from build123d import *

# Parameters (mm, degrees)
BOSS_EXTRUDE1_DEPTH = 6
FILLET1_R           = 1
FILLET2_R           = 0.5
SKETCH2_R           = 1.6
CUT_EXTRUDE2_DEPTH  = 10


with BuildPart() as part:
    # Sketch1 → Boss-Extrude1 (new body)
    with BuildSketch(Plane(origin=(0, 41.463460463, 0), x_dir=(1, 0, 0), z_dir=(0, 1, 0))):
        with BuildLine():
            Line((26.614370899, -46.171636097), (23.614370899, -38.171636097))
            Line((23.614370899, -38.171636097), (17.614370899, -38.171636097))
            Line((17.614370899, -38.171636097), (17.614370899, -35.202564725))
            Line((17.614370899, -35.202564725), (45.614370899, -35.202564725))
            Line((45.614370899, -35.202564725), (45.614370899, -38.171636097))
            Line((45.614370899, -38.171636097), (39.614370899, -38.171636097))
            Line((39.614370899, -38.171636097), (36.614370899, -46.171636097))
            ThreePointArc((36.614370899, -46.171636097), (31.614370899, -41.171636097), (26.614370899, -46.171636097))
        make_face()
    extrude(amount=-BOSS_EXTRUDE1_DEPTH)

    # Fillet1
    fillet1_edges = [part.edges().sort_by_distance(p)[0] for p in [
        (17.614370899, 41.463460463, 36.687100411),
        (45.614370899, 41.463460463, 36.687100411),
    ]]
    fillet(fillet1_edges, radius=FILLET1_R)

    # Fillet2
    fillet2_edges = [part.edges().sort_by_distance(p)[0] for p in [
        (36.614370899, 38.463460463, 46.171636097),
        (26.614370899, 38.463460463, 46.171636097),
    ]]
    fillet(fillet2_edges, radius=FILLET2_R)

    # Sketch2 → Cut-Extrude2 (cut)
    with BuildSketch(Plane(origin=(0, 0, 35.202564725), x_dir=(-1, 0, 0), z_dir=(0, 0, -1))):
        with Locations((-20.74213752, 38.663460463)):
            Circle(SKETCH2_R)
        with Locations((-42.486604277, 38.663460463)):
            Circle(SKETCH2_R)
    extrude(amount=-CUT_EXTRUDE2_DEPTH, mode=Mode.SUBTRACT)


solid = part.part
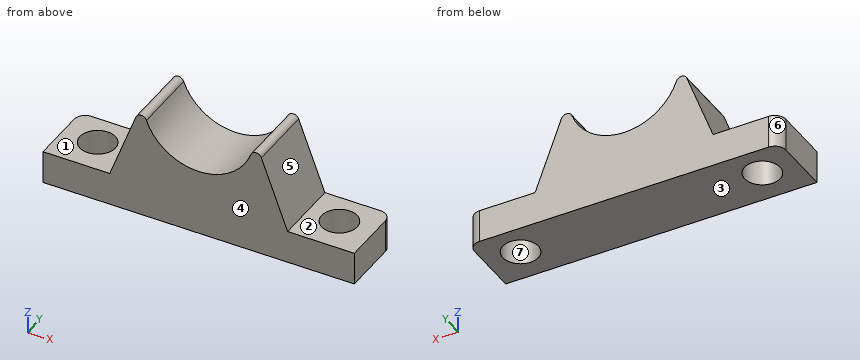
Here's how the part is built. I have some questions about the finished solid (model axes, mm). Face numbers are marked on the shaded views. A direction names the side the tool comes from. Round coordinates to 2 decimals unless told otherwise and drop trailing zeros. Write each loop counter-clockwise with the first axis right and the second up, starting at its lowest first coordinate (ties: lowest second). Pieces come first, ordered by that corner, then holes.
1. Suppose I cut it at C-C (y = 36.05). List the corners of the cut face in (x, z) for me, and give its area (3 significant figures).
2. Suppose I cut it at A-A (y = 39.55). List the corners of the cut face in (x, z) for me.
3. For the marked faces 1, 2 and 3, which set-ups out of +Z, -Z, +X, -X, +Y, -Y let a thin tool reach every point of the face, with its end or its side?
4. I need wall thicknesses on L1, parallel to X at y = 36.6, z = 42.25; L2, parallel to Y at x = 19.5, z = 37; L3, parallel to X at y = 37.95, z = 42.75. Which ranges of each line are inside material? Lowest first, please.
5. Will these pins go through, and if not, where does the flat tip stop? pin 1 Ø3 at (x, y) = (43, 38.5) entering from +Z; pin 2 Ø3 at (y, z) = (38.5, 40) entering from +X.
6. If we mould it in two halves opening along Y, with no side actions, what happens to the marked faces 4, 5, 6 and 7? For each: released by +Y, released by -Y, zero draft, split by the parting line, or undercut.
7. Suppose I cut it at B-B (x = 20.75). List the corners of the cut face in (y, z) for me, and give its area (3 significant figures).
8. Suppose I cut it at D-D (z = 41.5). List the corners of the cut face in (x, y) for me, and give its area (3 significant figures).
Answer sheet:
1. outline: (17.61, 35.2) - (45.61, 35.2) - (45.61, 38.17) - (39.61, 38.17) - (37.25, 44.47) arc R0.5 ccw to (36.31, 44.47) arc R5 cw to (26.91, 44.47) arc R0.5 ccw to (25.98, 44.47) - (23.61, 38.17) - (17.61, 38.17) - close
1. area: 147 mm2
2. outline: (17.61, 35.2) - (19.41, 35.2) - (19.41, 38.17) - (17.61, 38.17) - close; (22.07, 35.2) - (41.15, 35.2) - (41.15, 38.17) - (39.61, 38.17) - (37.25, 44.47) arc R0.5 ccw to (36.31, 44.47) arc R5 cw to (26.91, 44.47) arc R0.5 ccw to (25.98, 44.47) - (23.61, 38.17) - (22.07, 38.17) - close; (43.82, 35.2) - (45.61, 35.2) - (45.61, 38.17) - (43.82, 38.17) - close
3. face 1: +Z, -X, +Y, -Y
3. face 2: +Z, +X, +Y, -Y
3. face 3: -Z, +X, -X, +Y, -Y
4. L1: x = 25.14 to 28.51, 34.72 to 38.08
4. L2: y = 35.46 to 37.65, 39.67 to 41.46
4. L3: x = 25.33 to 27.97, 35.26 to 37.9
5. pin 1: stops at z = 38.17
5. pin 2: stops at x = 39.49
6. face 4: released by -Y
6. face 5: zero draft
6. face 6: released by +Y
6. face 7: undercut
7. outline: (35.46, 35.2) - (37.06, 35.2) - (37.06, 38.17) - (35.46, 38.17) - close; (40.26, 35.2) - (41.46, 35.2) - (41.46, 38.17) - (40.26, 38.17) - close
7. area: 8.31 mm2
8. outline: (24.86, 35.46) - (29.83, 35.46) - (29.83, 41.46) - (24.86, 41.46) - close; (33.4, 35.46) - (38.37, 35.46) - (38.37, 41.46) - (33.4, 41.46) - close
8. area: 59.6 mm2
